Check sheet for the modelled part. Datum: model origin and axes. Units: mm. Face numbers are marked on the shaded views. Round coordinates to 2 decimals unless told otherwise and drop trailing zeros. Write each loop counter-clockwise with the first axis right and the second up, starting at its lowest first coordinate (ties: lowest second). Pieces come first, ordered by that corner, then holes. Notation, with made-up numbers: (-8.5, 54.25) -> (5.5, 54.25) arc R14 ccw to (5.5, 72.25) -> close; hole circle Ø5 at (-39.5, -0.5). An arc over 180 degrees is marked (long way). Use one line per item in the form item = value. Start each with the question number.
```python
from build123d import *

# Parameters (mm, degrees)
SKETCH1_W           = 16
SKETCH1_H           = 20
BOSS_EXTRUDE1_DEPTH = 10
SKETCH2_R           = 2.25
CUT_EXTRUDE1_DEPTH  = 28.49545417
FILLET1_R           = 8
SKETCH3_W           = 16
SKETCH3_H           = 4.8
BOSS_EXTRUDE2_DEPTH = 10


with BuildPart() as part:
    # Sketch1 → Boss-Extrude1 (new body)
    with BuildSketch(Plane.XY):
        with Locations((8, 10)):
            Rectangle(SKETCH1_W, SKETCH1_H)
    extrude(amount=BOSS_EXTRUDE1_DEPTH)

    # Sketch2 → Cut-Extrude1 (cut, through all)
    with BuildSketch(Plane.XY.offset(10)):
        with Locations((8, 10.2)):
            Circle(SKETCH2_R)
    extrude(amount=-CUT_EXTRUDE1_DEPTH, mode=Mode.SUBTRACT)

    # Fillet1
    fillet1_edges = [part.edges().sort_by_distance(p)[0] for p in [
        (16, 20, 5),
        (0, 20, 5),
    ]]
    fillet(fillet1_edges, radius=FILLET1_R - 0.0001)  # a hair under: the kernel refuses the full size

    # Sketch3 → Boss-Extrude2 (add)
    with BuildSketch(Plane.XY.offset(10)):
        with Locations((8, -2.4)):
            Rectangle(SKETCH3_W, SKETCH3_H)
    extrude(amount=-BOSS_EXTRUDE2_DEPTH)


solid = part.part
```
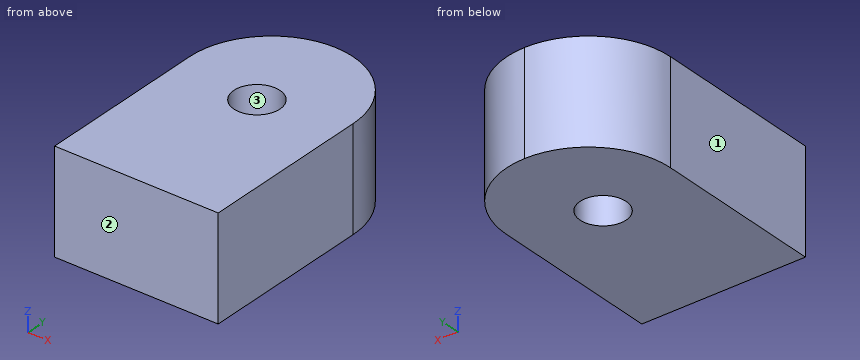
1. Sectioned sample at A-A (y = 10.2). Enter the section's corners in (x, z).
2. Mould release check, pull along Y, two halves, no side actions. Record for the marked faces 1, 2 and 3: +Y half, -Y half, draft (parallel to the pull), parting line (faces both ways), or undercut.
3. Depth check by flat-ended pin: pin 1 (3 mm diameter, centred on x = 12, y = 12, fed in from -Z). Enter the tip coordinate at first touch or a pass-through.
4. Sectioned sample at D-D (x = 1.5). Enter the section's corners in (y, z).
5. Sectioned sample at C-C (x = 7). Enter the section's corners in (y, z).
6. Scan lines: probe 1 along Y at (x, z) = (8, 6.5); probe 2 along X at (y, z) = (8.25, 9); probe 3 along X at (y, z) = (9.5, 3.5). Record each from-to range of solid material in increasing order.
Returned:
q1.outline = (0, 0) -> (5.75, 0) -> (5.75, 10) -> (0, 10) -> close; (10.25, 0) -> (16, 0) -> (16, 10) -> (10.25, 10) -> close
q2.face_1 = draft
q2.face_2 = -Y half
q2.face_3 = undercut
q3.pin_1 = 0
q4.outline = (-4.8, 0) -> (16.66, 0) -> (16.66, 10) -> (-4.8, 10) -> close
q5.outline = (-4.8, 0) -> (8.18, 0) -> (8.18, 10) -> (-4.8, 10) -> close; (12.22, 0) -> (19.94, 0) -> (19.94, 10) -> (12.22, 10) -> close
q6.probe_1 = -4.8 to 7.95, 12.45 to 20
q6.probe_2 = 0 to 6.88, 9.12 to 16
q6.probe_3 = 0 to 5.86, 10.14 to 16
